Here's how the part is built. I have some questions about the finished solid (model axes, mm). A direction names the side the tool comes from. Round coordinates to 2 decimals unless told otherwise and drop trailing zeros. Use a Markdown table: item, result. Add a question column.
```python
from build123d import *

# Parameters (mm, degrees)
SKETCH2_R                   = 39.2557
BOSS_EXTRUDE1_DEPTH         = 6.35
SKETCH4_R                   = 39.2557
SKETCH4_R_2                 = 36.5125
CUT_EXTRUDE1_DEPTH          = 3.175
F_1_4_0_25_DIAMETER_HOLE1_D = 6.35
F_1_2_0_5_DIAMETER_HOLE1_D  = 12.7
SKETCH9_R                   = 6.0325
CUT_EXTRUDE2_DEPTH          = 1.5875


with BuildPart() as part:
    # Sketch2 → Boss-Extrude1 (new body)
    with BuildSketch(Plane(origin=(0, 0, 0), x_dir=(1, 0, 0), z_dir=(0, 1, 0))):
        Circle(SKETCH2_R)
    extrude(amount=BOSS_EXTRUDE1_DEPTH)

    # Sketch4 → Cut-Extrude1 (cut)
    with BuildSketch(Plane(origin=(0, 6.35, 0), x_dir=(1, 0, 0), z_dir=(0, 1, 0))):
        Circle(SKETCH4_R)
        Circle(SKETCH4_R_2, mode=Mode.SUBTRACT)
    extrude(amount=-CUT_EXTRUDE1_DEPTH, mode=Mode.SUBTRACT)

    # 1/4 (0.25) Diameter Hole1 (through all)
    with Locations(Plane(origin=(0, 6.35, 0), x_dir=(1, 0, 0), z_dir=(0, 1, 0))):
        with Locations((-17.960512242, 17.960512242), (-17.960512242, -17.960512242), (17.960512242, 17.960512242), (17.960512242, -17.960512242)):
            Hole(F_1_4_0_25_DIAMETER_HOLE1_D / 2)

    # 1/2 (0.5) Diameter Hole1 (through all)
    with Locations(Plane(origin=(0, 6.35, 0), x_dir=(1, 0, 0), z_dir=(0, 1, 0))):
        with Locations((0, 0)):
            Hole(F_1_2_0_5_DIAMETER_HOLE1_D / 2)

    # Sketch9 → Cut-Extrude2 (cut)
    with BuildSketch(Plane.XZ):
        with Locations((-17.960512242, 17.960512242)):
            Circle(SKETCH9_R)
        with Locations((17.960512242, 17.960512242)):
            Circle(SKETCH9_R)
        with Locations((17.960512242, -17.960512242)):
            Circle(SKETCH9_R)
        with Locations((-17.960512242, -17.960512242)):
            Circle(SKETCH9_R)
    extrude(amount=-CUT_EXTRUDE2_DEPTH, mode=Mode.SUBTRACT)


solid = part.part
```
Item 1: If we mould it in two halves opening along Z, with no side actions, what happens to faces 4 (the face through (-20.99, 3.94, -18.91)), 5 (the face through (-28.933, 1.565, -26.531)), 6 (the face through (11, 3.175, 35))? For each: +Z half, -Z half, draft (parallel to the pull), parting line (faces both ways), or undercut.
Item 2: Imagine slicing it at C-C on z = 19. Count the separate pieces of the cut face and the enclosed holes in it, plus the area to 3 significant figures.
Item 3: On a 3-axis mill with a long thin cutter (end or side, diameter ignored), from which of +Z, -Z, +X, -X, +Y, -Y can I reach the whole of each face in a straight line? I mean faces 1 (the face through (21.132, 3.935, -18.1)), 2 (the face through (21.2, 0.78, -12.87)), 3 (the face through (34.826, 4.785, -10.967)). Say none if no direction works.
Item 4: I need wall thicknesses on probe 1 along Z at (x, y) = (-0.5, 1); probe 2 along Z at (x, y) = (19.5, 3); probe 3 along X at (y, z) = (6, 0.5). Which ranges of each line are inside material? Lowest first, please. Write a range as from..to.
Item 5: For pin 1 Ø5 at (x, z) = (17.96, -17.96) entering from +Y; pin 2 Ø9.5 at (x, z) = (17.96, 17.96) entering from -Y; pin 3 Ø2 at (x, y) = (-24.5, 1) entering from -Z; pin 4 Ø1.5 at (x, y) = (-3, 3.5) entering from +Z, each with a flat end and sliding along its axis, tell me the tip position at first contact or that it passes through.
The answers:
| question | item | result |
|---|---|---|
| 1 | face 4 | undercut |
| 1 | face 5 | parting line |
| 1 | face 6 | draft |
| 2 | separate pieces | 3 |
| 2 | enclosed holes | 0 |
| 2 | area | 321 mm² |
| 3 | face 1 | +Y, -Y |
| 3 | face 2 | -Y |
| 3 | face 3 | +Y |
| 4 | probe 1 | -39.25..-6.33, 6.33..39.25 |
| 4 | probe 2 | -34.07..-20.74, -15.18..15.18, 20.74..34.07 |
| 4 | probe 3 | -36.51..-6.33, 6.33..36.51 |
| 5 | pin 1 | through |
| 5 | pin 2 | y = 1.59 |
| 5 | pin 3 | z = -31.44 |
| 5 | pin 4 | z = 39.19 |
